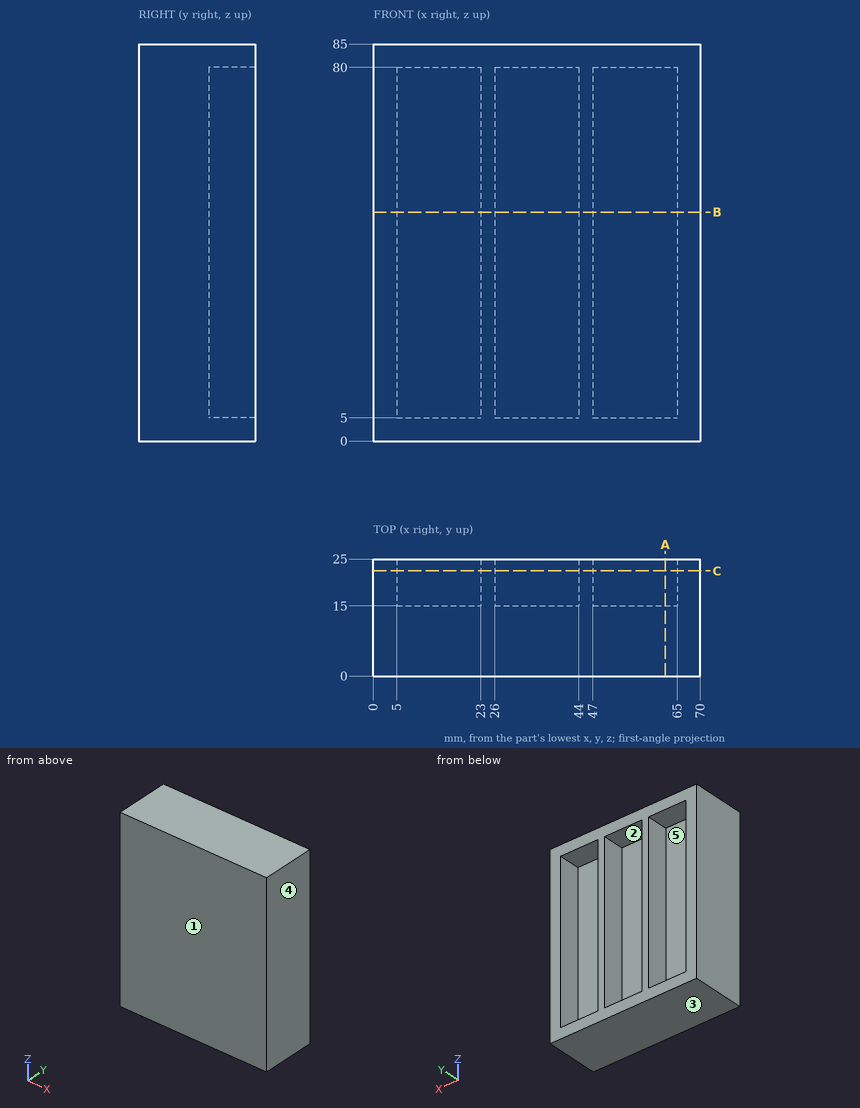
Verification items for this drawing (mm, ordinates from the low corner). A direction names the side the tool comes from. Round coordinates to 2 decimals unless told otherwise and drop trailing zeros. Order: outer loops, then holes, each group sorted by start corner. A loop starts at its lowest first (then second) coordinate and runs counter-clockwise, first axis right, second up. Notation, with made-up numbers: (59, 80.5) - (105, 80.5) arc R4 cw to (105, 84.5) - close; hole circle Ø6 at (38, -30.75). An arc over 180 degrees is marked (long way). Use CSV: the item, a comma, the result in double quotes. Start each with the question number.
1) Section check C-C, the plane y = 22.5. Record the cut outline in (x, z).
2) Go/stop test with a flat-tipped pin: P1, Ø1, axis at x = 35.5, z = 49.5, coming from the +Y side. Record where the tip stops, or that it passes through.
3) Thickness scan on L1, parallel to X at y = 21, z = 69; L2, parallel to Z at x = 34, y = 18.75; L3, parallel to Y at x = 38, z = 25. Record the ranges inside material, lowest first.
4) Mould release check, pull along X, two halves, no side actions. Record for the marked faces 3, 4 and 5: +X half, -X half, draft (parallel to the pull), parting line (faces both ways), or undercut.
5) Section check A-A, the plane x = 62.5. Record the cut outline in (y, z).
6) Access from +Z, -Z, +X, -X, +Y, -Y to the whole of each face (thin tool, end or side, straight path). Record for the marked faces 1 and 2.
7) Section check B-B, the plane z = 49. Record the cut outline in (x, y), plus the area to 3 significant figures.
Answers:
1,outline,"(0, 0) - (70, 0) - (70, 85) - (0, 85) - close; hole (5, 5) - (23, 5) - (23, 80) - (5, 80) - close; hole (26, 5) - (44, 5) - (44, 80) - (26, 80) - close; hole (47, 5) - (65, 5) - (65, 80) - (47, 80) - close"
2,P1,"stops at y = 15"
3,L1,"x = 0 to 5, 23 to 26, 44 to 47, 65 to 70"
3,L2,"z = 0 to 5, 80 to 85"
3,L3,"y = 0 to 15"
4,face 3,"draft"
4,face 4,"+X half"
4,face 5,"undercut"
5,outline,"(0, 0) - (25, 0) - (25, 5) - (15, 5) - (15, 80) - (25, 80) - (25, 85) - (0, 85) - close"
6,face 1,"+Z, -Z, +X, -X, -Y"
6,face 2,"+Y"
7,outline,"(0, 0) - (70, 0) - (70, 25) - (65, 25) - (65, 15) - (47, 15) - (47, 25) - (44, 25) - (44, 15) - (26, 15) - (26, 25) - (23, 25) - (23, 15) - (5, 15) - (5, 25) - (0, 25) - close"
7,area,"1,210 mm²"
